Build history of the part. All positions in model axes, mm. A direction names the side the tool comes from. Coordinates: 2 decimals unless noted, no trailing zeros. Loops run counter-clockwise (first coordinate to the right, second up) from the corner with the lowest first, then second, coordinate; pieces in that order, holes last.
(1) Slice it at B-B (z = 4.75). Give the cut face in (x, y).
(2) Slice it at C-C (y = -0.75). Give the cut face in (x, z), and give its area (3 significant figures).
(3) Slice it at D-D (y = 4). Give the cut face in (x, z), and give its area (3 significant figures).
(4) Slice it at A-A (x = 0). Give the cut face in (y, z), and give its area (3 significant figures).
(5) Tool access for faces 1 (the face through (-1, 2, 6)), 2 (the face through (-5.172, 3.042, 2.958)): list every direction of +Z, -Z, +X, -X, +Y, -Y with a clear straight run to the whole face (end or side of a thin tool).
(6) Two-plate mould, pull along X, no slides. Class faces 3 (the face through (-0.54, -2.44, 12.59)), 4 (the face through (0, 2, 3)), 5 (the face through (-2, 1, 0)), 6 (the face through (-5.22, -2.96, 2.96)): pulls with the +X half, pulls with the -X half, needs draft (parallel to the pull), parting line crosses it, or undercut.
(7) Wall check: L1, parallel to Y at x = 0, z = 1.9; L2, parallel to Y at x = 0, z = 9; L3, parallel to X at y = 2, z = 16.25. Give the ranges that are in metal, low to high.
(8) Flat gauge pins, fed straight in: P1, Ø2, axis at x = -1, z = 17, coming from the -Y side; P2, Ø2.5, axis at x = 0.5, y = -1, coming from the +Z side; P3, Ø2, axis at y = 3, z = 16.5, coming from the +X side; P4, Ø2, axis at x = -4, z = 2.5, coming from the +Y side. Where does each tip first touch, or does it go through?
from build123d import *

# Parameters (mm, degrees)
PAD_DEPTH       = 6
SKETCH001_R     = 5.5
PAD001_DEPTH    = 13
SKETCH002_R     = 2
POCKET_DEPTH    = 6
SKETCH003_R     = 2.5
POCKET001_DEPTH = 13


with BuildPart() as part:
    # Sketch → Pad (new body)
    with BuildSketch(Plane.XY):
        Polygon((6.928203, 0), (3.464102, 6), (-3.464102, 6), (-6.928203, 0), (-3.464102, -6), (3.464102, -6), align=None)
    extrude(amount=PAD_DEPTH)

    # Sketch001 (on Face8 of Pad) → Pad001 (join)
    with BuildSketch(Plane.XY.offset(6)):
        Circle(SKETCH001_R)
    extrude(amount=PAD001_DEPTH)

    # Sketch002 (on Face4 of Pad001) → Pocket (cut)
    with BuildSketch(Plane(origin=(0, 0, 0), x_dir=(1, 0, 0), z_dir=(0, 0, -1))):
        Circle(SKETCH002_R)
    extrude(amount=-POCKET_DEPTH, mode=Mode.SUBTRACT)

    # Sketch003 (on Face12 of Pocket) → Pocket001 (cut)
    with BuildSketch(Plane.XY.offset(19)):
        Circle(SKETCH003_R)
    extrude(amount=-POCKET001_DEPTH, mode=Mode.SUBTRACT)


solid = part.part
Response values:
1. outline: (-6.93, 0) - (-3.46, -6) - (3.46, -6) - (6.93, 0) - (3.46, 6) - (-3.46, 6) - close; hole circle Ø4 at (0, 0)
2. outline: (-6.5, 0) - (-1.85, 0) - (-1.85, 6) - (-2.38, 6) - (-2.38, 19) - (-5.45, 19) - (-5.45, 6) - (-6.5, 6) - close; (1.85, 0) - (6.5, 0) - (6.5, 6) - (5.45, 6) - (5.45, 19) - (2.38, 19) - (2.38, 6) - (1.85, 6) - close
2. area: 135 mm2
3. outline: (-4.62, 0) - (4.62, 0) - (4.62, 6) - (3.77, 6) - (3.77, 19) - (-3.77, 19) - (-3.77, 6) - (-4.62, 6) - close
3. area: 154 mm2
4. outline: (-6, 0) - (-2, 0) - (-2, 6) - (-2.5, 6) - (-2.5, 19) - (-5.5, 19) - (-5.5, 6) - (-6, 6) - close; (2, 0) - (6, 0) - (6, 6) - (5.5, 6) - (5.5, 19) - (2.5, 19) - (2.5, 6) - (2, 6) - close
4. area: 126 mm2
5. face 1: +Z
5. face 2: +Z, -Z, -X, +Y
6. face 3: undercut
6. face 4: undercut
6. face 5: needs draft
6. face 6: pulls with the -X half
7. L1: y = -6 to -2, 2 to 6
7. L2: y = -5.5 to -2.5, 2.5 to 5.5
7. L3: x = -5.12 to -1.5, 1.5 to 5.12
8. P1: stops at y = -5.5
8. P2: stops at z = 6
8. P3: stops at x = 5.12
8. P4: stops at y = 6
